Work out the finished part from the listing and answer in its coordinate system (mm). A direction names the side the tool comes from. Coordinates: 2 decimals unless noted, no trailing zeros. Write each loop counter-clockwise with the first axis right and the second up, starting at its lowest first coordinate (ties: lowest second). Pieces come first, ordered by that corner, then holes. Notation, with made-up numbers: (89, -35.5) - (99, -35.5) arc R16 cw to (99, -18.5) - close; hole circle Ø6 at (29.25, 51). An arc over 180 degrees is marked (long way). Use a Markdown table: item, result. Add a question column.
(1) A tool of negligible diameter and unlimited length cuts with its end or side. For faces 5 (the face through (0, 9, -26.772)), 6 (the face through (26.8, 16.5, -31.5)), 7 (the face through (-26.872, 16.441, -31.546)), from which of +Z, -Z, +X, -X, +Y, -Y can it reach the whole face along a straight path? Write none if from no direction.
(2) The part is cut by section D-D, the plane x = -16. Give the vertices of the cut face in (y, z), then the cut area to 3 significant figures.
(3) For a pull along Z with two mould halves and no side action, classify faces 1 (the face through (-2, 24, -29.032)), 2 (the face through (-27.864, 8.102, -31.745)), 3 (the face through (12, 11, -21)), 4 (the face through (19.203, 29.074, -32.252)) as released by +Z, released by -Z, zero draft, split by the parting line, or undercut.
(4) The part is cut by section A-A, the plane x = 0. Give the vertices of the cut face in (y, z), then the cut area to 3 significant figures.
(5) The part is cut by section B-B, the plane z = -21.5. Give the vertices of the cut face in (x, y).
(6) Given pin 1 Ø3 at (x, z) = (25, -13.5) entering from -Y; pin 2 Ø6 at (x, z) = (18.5, -6) entering from -Y; pin 3 Ø8 at (x, y) = (0, 29.11) entering from +Z; pin 4 Ø1.5 at (x, z) = (-13, -23.5) entering from +Y, each flat-ended and moving along its own axis, determine where each tip first touches the part or whether it passes through.
(7) The part is cut by section C-C, the plane y = 39.5. Give the vertices of the cut face in (x, z).
(8) Find the intervals of material crossed by line 1 (Z direction, x = -12, y = 32); line 2 (X direction, y = 13.5, z = -20); line 3 (X direction, y = 10, z = -16), in increasing order. Write a range as from..to.
from build123d import *

# Parameters (mm, degrees)
BOSS_EXTRUDE1_DEPTH             = 43.18
CUT_EXTRUDE1_DEPTH              = 27.94
SKETCH6_W                       = 92.402659054
SKETCH6_H                       = 40.294164386
CUT_EXTRUDE3_DEPTH              = 25.4
TAP_DRILL_FOR_M8X1_0_TAP1_D     = 7
TAP_DRILL_FOR_M8X1_0_TAP1_DEPTH = 8.001
TAP_DRILL_FOR_M8X1_0_TAP1_TIP   = 2.103012167
CUT_EXTRUDE4_DEPTH              = 12.7
CUT_EXTRUDE5_DEPTH              = 15.24
F_3_8_CLEARANCE_HOLE1_D         = 10.0838
F_3_8_CLEARANCE_HOLE1_DEPTH     = 35.941
F_3_8_CLEARANCE_HOLE1_TIP       = 3.029479155
CUT_EXTRUDE6_DEPTH              = 15.24
CUT_EXTRUDE7_DEPTH              = 15.24
FILLET2_R                       = 12.7
FILLET3_R                       = 5.08
FILLET5_R                       = 5.08
FILLET4_R                       = 12.7
SKETCH16_W                      = 36.875028965
SKETCH16_H                      = 42.723051179
CUT_EXTRUDE8_DEPTH              = 12.7
SKETCH18_W                      = 36.753195168
SKETCH18_H                      = 42.885496241
CUT_EXTRUDE9_DEPTH              = 12.7
CUT_EXTRUDE10_DEPTH             = 65.85933151
CUT_EXTRUDE10_DEPTH_BACK        = 65.85933151


with BuildPart() as part:
    # Sketch1 → Boss-Extrude1 (new body)
    with BuildSketch(Plane(origin=(0, 0, 0), x_dir=(1, 0, 0), z_dir=(0, 1, 0))):
        Polygon((-26.9367, 35.3822), (26.9367, 35.3822), (44.45, 0), (-44.45, 0), align=None)
    extrude(amount=BOSS_EXTRUDE1_DEPTH)

    # Sketch3 → Cut-Extrude1 (cut)
    with BuildSketch(Plane(origin=(0, 43.18, 0), x_dir=(1, 0, 0), z_dir=(0, 1, 0))):
        Polygon((-30.079790452, 29.0322), (30.079790452, 29.0322), (41.306909548, 6.35), (-41.306909548, 6.35), align=None)
    extrude(amount=-CUT_EXTRUDE1_DEPTH, mode=Mode.SUBTRACT)

    # Sketch6 → Cut-Extrude3 (cut)
    with BuildSketch(Plane(origin=(0, 11.371619882, -4.138931152), x_dir=(-1, 0, 0), z_dir=(0, -0.939692620785908, 0.34202014332566977))):
        with Locations((0.08638911, 14.200910291)):
            Rectangle(SKETCH6_W, SKETCH6_H)
    extrude(amount=CUT_EXTRUDE3_DEPTH, mode=Mode.SUBTRACT)

    # Tap Drill for M8x1.0 Tap1
    with Locations(Plane(origin=(0, 11.371619882, -4.138931152), x_dir=(-1, 0, 0), z_dir=(0, -0.939692620785908, 0.3420201433256697))):
        with Locations((22.225, 8.988861466), (-22.225, 8.988861466)):
            Hole(TAP_DRILL_FOR_M8X1_0_TAP1_D / 2, depth=TAP_DRILL_FOR_M8X1_0_TAP1_DEPTH)
            with Locations((0, 0, -(TAP_DRILL_FOR_M8X1_0_TAP1_DEPTH + TAP_DRILL_FOR_M8X1_0_TAP1_TIP / 2))):  # 118° drill point
                Cone(0, TAP_DRILL_FOR_M8X1_0_TAP1_D / 2, TAP_DRILL_FOR_M8X1_0_TAP1_TIP, mode=Mode.SUBTRACT)

    # Sketch10 → Cut-Extrude4 (cut)
    with BuildSketch(Plane(origin=(0, 15.24, -4.821030939), x_dir=(1, 0, 0), z_dir=(0, -1, 0))):
        with BuildLine():
            Line((-4.1275, -5.440569061), (4.1275, -5.440569061))
            ThreePointArc((4.1275, -5.440569061), (12.3825, -13.695569061), (4.1275, -21.950569061))
            Line((4.1275, -21.950569061), (-4.1275, -21.950569061))
            ThreePointArc((-4.1275, -21.950569061), (-12.3825, -13.695569061), (-4.1275, -5.440569061))
        make_face()
    extrude(amount=CUT_EXTRUDE4_DEPTH, mode=Mode.SUBTRACT)

    # Sketch11 → Cut-Extrude5 (cut)
    with BuildSketch(Plane(origin=(0, 11.371619882, -4.138931152), x_dir=(1, 0, 0), z_dir=(0, -0.939692620785908, 0.3420201433256697))):
        Polygon((-26.9367, -33.248392247), (26.9367, -33.248392247), (29.430898409, -27.885957416), (-29.430898409, -27.885957416), align=None)
    extrude(amount=-CUT_EXTRUDE5_DEPTH, mode=Mode.SUBTRACT)

    # 3/8 Clearance Hole1
    with Locations(Plane(origin=(0, 0, -35.3822), x_dir=(-1, 0, 0), z_dir=(0, 0, -1))):
        with Locations((0, 29.1084)):
            Hole(F_3_8_CLEARANCE_HOLE1_D / 2, depth=F_3_8_CLEARANCE_HOLE1_DEPTH)
            with Locations((0, 0, -(F_3_8_CLEARANCE_HOLE1_DEPTH + F_3_8_CLEARANCE_HOLE1_TIP / 2))):  # 118° drill point
                Cone(0, F_3_8_CLEARANCE_HOLE1_D / 2, F_3_8_CLEARANCE_HOLE1_TIP, mode=Mode.SUBTRACT)

    # Sketch14 → Cut-Extrude6 (cut)
    with BuildSketch(Plane(origin=(0, 0, -35.3822), x_dir=(-1, 0, 0), z_dir=(0, 0, -1))):
        Polygon((-26.9367, 15.678710556), (-11.058823136, 43.18), (-30.079790452, 43.18), (-30.079790452, 15.24), align=None)
        Polygon((26.9367, 15.678710556), (11.058823136, 43.18), (30.079790452, 43.18), (30.079790452, 15.24), align=None)
    extrude(amount=-CUT_EXTRUDE6_DEPTH, mode=Mode.SUBTRACT)

    # Sketch15 → Cut-Extrude7 (cut)
    with BuildSketch(Plane(origin=(0, 0, -6.35), x_dir=(-1, 0, 0), z_dir=(0, 0, -1))):
        Polygon((-41.306909548, 15.24), (-17.862465853, 43.18), (-44.45, 43.18), (-44.45, 12.878067623), align=None)
        Polygon((41.306909548, 15.24), (17.862465853, 43.18), (44.45, 43.18), (44.45, 12.878067623), align=None)
    extrude(amount=-CUT_EXTRUDE7_DEPTH, mode=Mode.SUBTRACT)

    # Fillet2
    # the kernel refuses this fillet: 12.7 mm, written as the material it adds along each edge
    with BuildSketch(Plane(origin=(41.306909548, 15.24, -6.35), x_dir=(0.7994362738246867, -0.6007509002018228, 0), z_dir=(0, 0, 1))) as fillet2_piece_1_section:
        with BuildLine():
            CenterArc((FILLET2_R * 0.114610182793, FILLET2_R), FILLET2_R, 256.923695862, 13.076304138)
            Line((-FILLET2_R * 0.111638297241, FILLET2_R * 0.0259303796532), (0, 0))
            Line((0, 0), (FILLET2_R * 0.114610182793, 0))
        make_face()
    fillet2_piece_1 = extrude(amount=6.35, mode=Mode.PRIVATE)
    fillet2_piece_1 = split(fillet2_piece_1, bisect_by=Plane(origin=(42.634214794, 15.269843294, -3.668439147), z_dir=(-0.8962213844521023, 0, 0.4436070671785529)), keep=Keep.TOP, mode=Mode.PRIVATE)
    add(fillet2_piece_1)
    with BuildSketch(Plane(origin=(-41.306909548, 15.24, -6.35), x_dir=(-0.7994362738246867, -0.6007509002018229, 0), z_dir=(0, 0, 1))) as fillet2_piece_2_section:
        with BuildLine():
            CenterArc((FILLET2_R * 0.114610182793, -FILLET2_R), FILLET2_R, 90, 13.076304138)
            Line((-FILLET2_R * 0.111638297241, -FILLET2_R * 0.0259303796532), (0, 0))
            Line((0, 0), (FILLET2_R * 0.114610182793, 0))
        make_face()
    fillet2_piece_2 = extrude(amount=6.35, mode=Mode.PRIVATE)
    fillet2_piece_2 = split(fillet2_piece_2, bisect_by=Plane(origin=(-42.634214794, 15.269843294, -3.668439147), z_dir=(0.8962213844521023, 0, 0.4436070671785529)), keep=Keep.TOP, mode=Mode.PRIVATE)
    add(fillet2_piece_2)
    # the kernel refuses this fillet: 12.7 mm, written as the material it takes off along each edge
    with BuildSketch(Plane(origin=(17.862465853, 43.18, -21.155268146), x_dir=(-1, 0, 0), z_dir=(0, 0, 1)), Plane(origin=(-17.862465853, 43.18, -21.155268146), x_dir=(-0.6427876096865353, -0.7660444431189815, 0), z_dir=(0, 0, 1))) as fillet2_2_piece_1:
        with BuildLine():
            CenterArc((FILLET2_R * 0.466307658155, FILLET2_R), FILLET2_R, 220, 50)
            Line((-FILLET2_R * 0.299736784964, FILLET2_R * 0.357212390313), (0, 0))
            Line((0, 0), (FILLET2_R * 0.466307658155, 0))
        make_face()
    extrude(amount=35.960536293, mode=Mode.SUBTRACT)

    # Fillet3
    # the kernel refuses this fillet: 5.08 mm, written as the material it adds along each edge
    with BuildSketch(Plane(origin=(26.9367, 15.678710556, -35.3822), x_dir=(0.9903988653234791, -0.1382392403262007, 0), z_dir=(0, 0, 1))) as fillet3_piece_1_section:
        with BuildLine():
            CenterArc((FILLET3_R * 0.488316369793, FILLET3_R), FILLET3_R, 217.945971462, 52.054028538)
            Line((-FILLET3_R * 0.300274587293, FILLET3_R * 0.385081873416), (0, 0))
            Line((0, 0), (FILLET3_R * 0.488316369793, 0))
        make_face()
    fillet3_piece_1 = extrude(amount=6.35, mode=Mode.PRIVATE)
    fillet3_piece_1 = split(fillet3_piece_1, bisect_by=Plane(origin=(28.34322893, 16.154895704, -32.540583178), z_dir=(-0.8962213844519045, 0, 0.4436070671789527)), keep=Keep.TOP, mode=Mode.PRIVATE)
    add(fillet3_piece_1)
    with BuildSketch(Plane(origin=(-26.9367, 15.678710556, -35.3822), x_dir=(-0.9903988653234792, -0.13823924032619928, 0), z_dir=(0, 0, 1))) as fillet3_piece_2_section:
        with BuildLine():
            CenterArc((FILLET3_R * 0.488316369793, -FILLET3_R), FILLET3_R, 90, 52.054028538)
            Line((-FILLET3_R * 0.300274587293, -FILLET3_R * 0.385081873416), (0, 0))
            Line((0, 0), (FILLET3_R * 0.488316369793, 0))
        make_face()
    fillet3_piece_2 = extrude(amount=6.35, mode=Mode.PRIVATE)
    fillet3_piece_2 = split(fillet3_piece_2, bisect_by=Plane(origin=(-28.34322893, 16.154895704, -32.540583178), z_dir=(0.8962213844519045, 0, 0.4436070671789527)), keep=Keep.TOP, mode=Mode.PRIVATE)
    add(fillet3_piece_2)
    # the kernel refuses this fillet: 5.08 mm, written as the material it takes off along each edge
    with BuildSketch(Plane(origin=(11.058823136, 43.18, -42.714548419), x_dir=(0.49999999999999484, -0.8660254037844416, 0), z_dir=(0, 0, 1)), Plane(origin=(-11.058823136, 43.18, -42.714548419), x_dir=(1, 0, 0), z_dir=(0, 0, 1))) as fillet3_2_piece_1:
        with BuildLine():
            CenterArc((FILLET3_R * 0.57735026919, -FILLET3_R), FILLET3_R, 90, 60)
            Line((-FILLET3_R * 0.288675134595, -FILLET3_R * 0.5), (0, 0))
            Line((0, 0), (FILLET3_R * 0.57735026919, 0))
        make_face()
    extrude(amount=21.014696837, mode=Mode.SUBTRACT)

    # Fillet5
    fillet5_edges = [part.edges().sort_by_distance(p)[0] for p in [
        (28.183799204, 8.756385643, -32.86267978),
        (-28.183799204, 8.756385643, -32.86267978),
    ]]
    fillet(fillet5_edges, radius=FILLET5_R)

    # Fillet4
    # the kernel refuses this fillet: 12.7 mm, written as the material it takes off along each edge
    with BuildSketch(Plane(origin=(-29.229670418, 15.678710556, -35.3822), x_dir=(0, 1, 0), z_dir=(1, 0, 0))) as fillet4_piece_1:
        with BuildLine():
            CenterArc((FILLET4_R * 0.176326980708, FILLET4_R), FILLET4_R, 250, 20)
            Line((-FILLET4_R * 0.165693162617, FILLET4_R * 0.0603073792141), (0, 0))
            Line((0, 0), (FILLET4_R * 0.176326980708, 0))
        make_face()
    extrude(amount=58.459340836, mode=Mode.SUBTRACT)

    # Sketch16 → Cut-Extrude8 (cut)
    with BuildSketch(Plane(origin=(-45.72, 0, 0), x_dir=(0, 0, -1), z_dir=(1, 0, 0))):
        with Locations((17.528654939, 22.385196569)):
            Rectangle(SKETCH16_W, SKETCH16_H)
    extrude(amount=CUT_EXTRUDE8_DEPTH, mode=Mode.SUBTRACT)

    # Sketch18 → Cut-Extrude9 (cut)
    with BuildSketch(Plane.ZY.offset(-45.72)):
        with Locations((-17.752016898, 22.669475427)):
            Rectangle(SKETCH18_W, SKETCH18_H)
    extrude(amount=CUT_EXTRUDE9_DEPTH, mode=Mode.SUBTRACT)

    # Sketch19 → Cut-Extrude10 (cut, two sides: drawn at the far end of the back side and taken through both)
    with BuildSketch(Plane(origin=(0, 0, 0), x_dir=(0, 0, -1), z_dir=(1, 0, 0)).offset(-CUT_EXTRUDE10_DEPTH_BACK)):
        Polygon((29.0322, 43.18), (35.3822, 40.868789012), (35.3822, 43.18), align=None)
    extrude(amount=CUT_EXTRUDE10_DEPTH + CUT_EXTRUDE10_DEPTH_BACK, mode=Mode.SUBTRACT)


solid = part.part
Model answer:
| question | item | result |
|---|---|---|
| 1 | face 5 | +Y, -Y |
| 1 | face 6 | -Z, +X, +Y |
| 1 | face 7 | -Z, -X, +Y |
| 2 | outline | (1.83, -30.34) - (13.57, -34.62) arc R12.7 ccw to (17.92, -35.38) - (34.62, -35.38) - (34.62, -29.03) - (15.24, -29.03) - (15.24, -6.35) - (42.51, -6.35) - (42.51, 0) - (12.88, 0) - close |
| 2 | area | 568 mm^2 |
| 3 | face 1 | undercut |
| 3 | face 2 | released by -Z |
| 3 | face 3 | undercut |
| 3 | face 4 | zero draft |
| 4 | outline | (1.83, -30.34) - (13.57, -34.62) arc R12.7 ccw to (17.92, -35.38) - (24.07, -35.38) - (24.07, -29.03) - (15.24, -29.03) - (15.24, -26.77) - (3.13, -26.77) - close; (9.14, -10.26) - (15.24, -10.26) - (15.24, -6.35) - (24.07, -6.35) - (24.07, 0) - (12.88, 0) - close; (34.15, -35.38) - (40.87, -35.38) - (43.18, -29.03) - (34.15, -29.03) - close; (34.15, -6.35) - (43.18, -6.35) - (43.18, 0) - (34.15, 0) - close |
| 4 | area | 341 mm^2 |
| 5 | outline | (-33.02, 5.05) - (-11.82, 5.05) - (-11.82, 15.24) - (-33.02, 15.24) - close; (11.82, 5.05) - (33.02, 5.05) - (33.02, 15.24) - (11.82, 15.24) - close |
| 6 | pin 1 | y = 7.42 |
| 6 | pin 2 | y = 9.6 |
| 6 | pin 3 | through |
| 6 | pin 4 | y = 15.24 |
| 7 | outline | (-20.88, -6.35) - (20.88, -6.35) - (20.88, 0) - (-20.88, 0) - close; (-13.18, -35.38) - (13.18, -35.38) - (13.18, -29.03) - (-13.18, -29.03) - close |
| 8 | line 1 | -35.38..-29.03, -6.35..0 |
| 8 | line 2 | -33.02..-12.25, 12.25..33.02 |
| 8 | line 3 | -33.02..-24.54, -19.91..-11.99, 11.99..19.91, 24.54..33.02 |
